Geometry: see drawing. Coordinates: mm, zero at the bounding-box minimum. Give positions to 0.01 mm unless a question says otherwise; leave off trailing zeros. Order: outer loops, then holes, each group sorted by start corner. A loop starts at its lowest first (then second) coordinate and runs counter-clockwise, first axis right, second up. Notation, with made-up numbers: M 59.25,48 L 113.25,48 A9 ccw 113.25,56 Z; hole C 42.5,-31.75 d7. An arc over 180 degrees is marked long. Return JSON: item names as keys, results as strings.
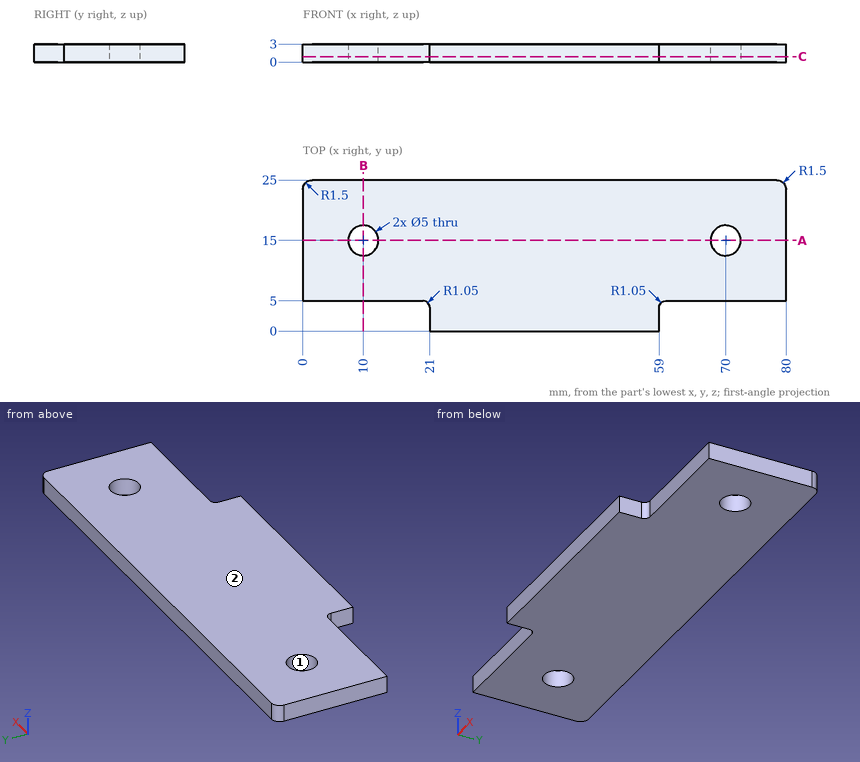
1. Ray query, probe 1 along Y at (x, z) = (10, 0.7); probe 2 along X at (y, z) = (16.5, 2); probe 3 along Y at (x, z) = (69, 1.85). Return the intervals inside material, ascending.
Evaluation:
{"probe 1": "y = 5 to 12.5, 17.5 to 25", "probe 2": "x = 0 to 8, 12 to 68, 72 to 80", "probe 3": "y = 5 to 12.71, 17.29 to 25"}
2. Section query B-B (x = 10). Return loops of the section in (y, z), then the cut area to 3 significant figures.
Evaluation:
{"outline": "M 5,0 L 12.5,0 L 12.5,3 L 5,3 Z; M 17.5,0 L 25,0 L 25,3 L 17.5,3 Z", "area": "45.0 mm^2"}
3. Section query C-C (z = 0.9). Return loops of the section in (x, y).
Evaluation:
{"outline": "M 0,5 L 19.95,5 A1.05 cw 21,3.95 L 21,0 L 59,0 L 59,3.95 A1.05 cw 60.05,5 L 80,5 L 80,23.5 A1.5 ccw 78.5,25 L 1.5,25 A1.5 ccw 0,23.5 Z; hole C 10,15 d5; hole C 70,15 d5"}
4. First-contact query: pin 1 (1.5 mm diameter, centred on x = 69.5, z = 1, fed in from -Y). Flat tip, straight axial feed; report the tip coordinate or a pass-through.
Evaluation:
{"pin 1": "stops at y = 5"}
5. Section query A-A (y = 15). Return loops of the section in (x, z).
Evaluation:
{"outline": "M 0,0 L 7.5,0 L 7.5,3 L 0,3 Z; M 12.5,0 L 67.5,0 L 67.5,3 L 12.5,3 Z; M 72.5,0 L 80,0 L 80,3 L 72.5,3 Z"}
6. Draft query along Y for the marked faces 1 and 2. Return one class per face: pulls with the +Y half, pulls with the -Y half, needs draft (parallel to the pull), parting line crosses it, or undercut.
Evaluation:
{"face 1": "undercut", "face 2": "needs draft"}
